from build123d import *

# Parameters (mm, degrees)
BOSS_EXTRUDE1_DEPTH = 6.35
LPATTERN1_COUNT     = 3
LPATTERN1_PITCH     = 31.75
LPATTERN2_COUNT     = 3
LPATTERN2_PITCH     = 25.4
FILLET1_R           = 3.81


with BuildPart() as part:
    # Sketch1 → Boss-Extrude1 (new, symmetric)
    with BuildSketch(Plane.XY):
        Polygon((0, 0), (-88.9, 0), (-88.9, -12.7), (-12.7, -82.55), (0, -82.55), align=None)
    extrude(amount=BOSS_EXTRUDE1_DEPTH, both=True)

    # Sketch3 → Tap Drill for 1/4-20 Tap1 (revolve, cut)
    with BuildSketch(Plane(origin=(-76.2, 0, 0), x_dir=(0, 0, 1), z_dir=(1, 0, 0))):
        Polygon((0, 0), (0, 14.233816902), (2.5527, 12.7), (2.5527, 0), align=None)
    tap_drill_for_1_4_20_tap1 = revolve(axis=Axis((-76.2, 6.35, 0), (0, -1, 0)), mode=Mode.SUBTRACT)

    # LPattern1: Tap Drill for 1/4-20 Tap1 ×3
    with Locations(*[(i * LPATTERN1_PITCH, 0, 0) for i in range(1, LPATTERN1_COUNT)]):
        add(tap_drill_for_1_4_20_tap1, mode=Mode.SUBTRACT)

    # Sketch5 → Tap Drill for 1/4-20 Tap2 (revolve, cut)
    with BuildSketch(Plane(origin=(0, -69.85, 0), x_dir=(0, 0, -1), z_dir=(0, 1, 0))):
        Polygon((0, 0), (0, 14.233816902), (2.5527, 12.7), (2.5527, 0), align=None)
    tap_drill_for_1_4_20_tap2 = revolve(axis=Axis((6.35, -69.85, 0), (-1, 0, 0)), mode=Mode.SUBTRACT)

    # LPattern2: Tap Drill for 1/4-20 Tap2 ×3
    with Locations(*[(0, i * LPATTERN2_PITCH, 0) for i in range(1, LPATTERN2_COUNT)]):
        add(tap_drill_for_1_4_20_tap2, mode=Mode.SUBTRACT)

    # Fillet1
    fillet1_edges = [part.edges().sort_by_distance(p)[0] for p in [
        (-12.7, -82.55, 0),
        (-88.9, -12.7, 0),
    ]]
    fillet(fillet1_edges, radius=FILLET1_R)


solid = part.part
CAD build for the part. Positions are in the model's coordinates, mm. A direction names the side the tool comes from. Coordinates: 2 decimals unless noted, no trailing zeros. Write each loop counter-clockwise with the first axis right and the second up, starting at its lowest first coordinate (ties: lowest second). Pieces come first, ordered by that corner, then holes. Notation, with made-up numbers: (75, 64) - (87, 64) arc R27 cw to (87, 97) - close; hole circle Ø11 at (-39, 89.25). An arc over 180 degrees is marked (long way). Use a Markdown table: item, result. Add a question column.
Item 1: Drill centre lines: L1, parallel to X at y = -4, z = 0; L2, parallel to Y at x = -8.5, z = 0; L3, parallel to X at y = -10.5, z = 0.75. Where is each one in solid material? Low to high. Write a range as from..to.
Item 2: Band-saw the part on D-D, the plane y = -65. Give the cut face in (x, z), and give its area (3 significant figures).
Item 3: Band-saw the part on C-C, the plane x = -40. Give the cut face in (y, z) (3 decimals).
Item 4: Flat gauge pins, fed straight in: pin 1 (6.5 mm diameter, centred on x = -76.2, z = 0, fed in from -Y); pin 2 (4.5 mm diameter, centred on x = -44.45, z = 0, fed in from -Y); pin 3 (4 mm diameter, centred on y = -44.45, z = 0, fed in from -X). Where does each tip first touch, or does it go through?
Item 5: 3-axis set-ups, long thin cutter, end or side, ignore diameter. For faces 4 (the face through (-6.26, -72.38, 0.33)), 5 (the face through (-15.23, -6.26, -0.33)), 6 (the face through (-44, 0, -3)): which of +Z, -Z, +X, -X, +Y, -Y reach the whole face in a straight line?
Item 6: Band-saw the part on B-B, the plane z = 4. Give the cut face in (x, y).
Item 7: Band-saw the part on A-A, the plane y = -10. Give the cut face in (x, z).
Item 8: Mould opens along X. For faces 1 (the face through (-13.97, -44.02, 0.1)), 2 (the face through (-35, -32, -6.35)), 3 (the face through (-44.02, -13.97, -0.1)) say: pulls with the +X half, pulls with the -X half, needs draft (parallel to the pull), parting line crosses it, or undercut.
Numbers:
| question | item | result |
|---|---|---|
| 1 | L1 | -88.9..-78.75, -73.65..-47, -41.9..-15.25, -10.15..0 |
| 1 | L2 | -82.55..-72.4, -67.3..-47, -41.9..-21.6, -16.5..0 |
| 1 | L3 | -88.9..-78.64, -73.76..-46.89, -42.01..-15.14, -10.26..0 |
| 2 | outline | (-31.85, -6.35) - (0, -6.35) - (0, 6.35) - (-31.85, 6.35) - close |
| 2 | area | 404 mm2 |
| 3 | outline | (-57.525, -6.35) - (0, -6.35) - (0, 6.35) - (-57.525, 6.35) - close |
| 4 | pin 1 | y = -27.32 |
| 4 | pin 2 | y = -55.51 |
| 4 | pin 3 | x = -56.45 |
| 5 | face 4 | +X |
| 5 | face 5 | +Y |
| 5 | face 6 | +Z, -Z, +X, -X, +Y |
| 6 | outline | (-88.9, -11.02) arc R3.81 ccw to (-87.66, -13.83) - (-13.79, -81.55) arc R3.81 ccw to (-11.22, -82.55) - (0, -82.55) - (0, 0) - (-88.9, 0) - close |
| 7 | outline | (-88.9, -6.35) - (0, -6.35) - (0, 6.35) - (-88.9, 6.35) - close; hole circle Ø5.11 at (-76.2, 0); hole circle Ø5.11 at (-44.45, 0); hole circle Ø5.11 at (-12.7, 0) |
| 8 | face 1 | pulls with the +X half |
| 8 | face 2 | needs draft |
| 8 | face 3 | undercut |
